Autodesk Inventor part; units mm, degrees
ref_plane "YZ Plane" through (0, 0, 0) normal (1, 0, 0) x (0, 1, 0)
ref_plane "XZ Plane" through (0, 0, 0) normal (0, 1, 0) x (-1, 0, 0)
ref_plane "XY Plane" through (0, 0, 0) normal (0, 0, 1) x (1, 0, 0)
sketch "Sketch1" plane through (0, 0, 0) normal (0, 0, 1) x (1, 0, 0)
  line L0 (-2, 0) -> (2, 0)
  line L1 (-2, 0) -> (-2, 3)
  line L2 (-2, 3) -> (-1.9, 3)
  line L3 (0, 0) -> (0, 3) construction
  line L4 (-1.9, 3) -> (-1.9, 3.6)
  line L5 (-1.5, 4) -> (-1.3196, 4)
  line L6 (-0.9732, 3.8) -> (-0.6268, 3.2)
  line L7 (-0.2804, 3) -> (0, 3)
  arc A0 (-0.9732, 3.8) -> (-1.3196, 4) centre (-1.3196, 3.6) ccw
  arc A1 (-0.6268, 3.2) -> (-0.2804, 3) centre (-0.2804, 3.4) ccw
  arc A2 (-1.5, 4) -> (-1.9, 3.6) centre (-1.5, 3.6) ccw
  line L8 (2, 0) -> (2, 3)
  line L9 (2, 3) -> (1.9, 3)
  line L10 (1.9, 3) -> (1.9, 3.6)
  line L11 (1.5, 4) -> (1.3196, 4)
  line L12 (0.9732, 3.8) -> (0.6268, 3.2)
  line L13 (0.2804, 3) -> (0, 3)
  arc A3 (1.3196, 4) -> (0.9732, 3.8) centre (1.3196, 3.6) ccw
  arc A4 (0.2804, 3) -> (0.6268, 3.2) centre (0.2804, 3.4) ccw
  arc A5 (1.9, 3.6) -> (1.5, 4) centre (1.5, 3.6) ccw
  line L14 (-0.8, 3.5) -> (0.8, 3.5) construction
  dimension "d0" = 0.4
  dimension "d1" = 8
  dimension "d2" = 6
  dimension "d3" = 6
  dimension "d4" = 4
  dimension "d5" = 3.8
  dimension "d8" = 1.6
  dimension "d9" = 120
revolve "Revolution1" add sketch "Sketch1" angle 360 about axis through (-2, 0, 0) along (1, 0, 0)
sketch "Sketch2" plane through (2, 0, 0) normal (1, 0, 0) x (0, 0, -1)
  circle A0 centre (0, 0) radius 2.5
  line L0 (2.2405, -1.1091) -> (1.6314, -0.5) construction
  line L1 (1.1314, 0) -> (1.6314, 0.5)
  line L2 (-2.2405, 1.1091) -> (-1.6314, 0.5) construction
  line L3 (-1.1314, 0) -> (-1.6314, -0.5)
  line L4 (-1.1091, -2.2405) -> (0, -1.1314)
  line L5 (0, -1.1314) -> (1.1091, -2.2405)
  line L6 (1.1091, 2.2405) -> (0, 1.1314)
  line L7 (0, 1.1314) -> (-1.1091, 2.2405)
  line L8 (-1.6314, -0.5) -> (-2.4495, -0.5)
  line L9 (-1.6314, 0.5) -> (-2.4495, 0.5)
  line L10 (1.6314, -0.5) -> (2.4495, -0.5)
  line L11 (1.6314, 0.5) -> (2.4495, 0.5)
  line L12 (-1.6314, -0.5) -> (-2.2405, -1.1091) construction
  line L13 (1.6314, -0.5) -> (1.1314, 0)
  line L14 (1.6314, 0.5) -> (2.2405, 1.1091) construction
  line L15 (-1.6314, 0.5) -> (-1.1314, 0)
  point P0 (0, 0)
  dimension "d11" = 5
  dimension "d12" = 1.6
  dimension "d13" = 1
  dimension "d14" = 1
  dimension "d15" = 1.5685
  dimension "d16" = 1.5685
  dimension "d17" = 1.6
  dimension "d18" = 1.6
  dimension "d19" = 1.6
extrude "Extrusion1" cut sketch "Sketch2" against normal through all contours L11 L1 L13 L10 A0 L5 L4 L8 L3 L15 L9 L7 L6
fillet "Fillet1" radius 0.3 6 edges at (0, 0, 1.1314) (0, 0.5, 1.6314) (0, -0.5, 1.6314) (0, 0.5, -1.6314) (0, 0, -1.1314) (0, -0.5, -1.6314)
fillet "Fillet2" radius 0.8 2 edges at (0, -1.1314, 0) (0, 1.1314, 0)
equation "\"d3\" = d2"
equation "\"d14\" = d13"
equation "\"d16\" = d15"
equation "\"d17\" = d12"
equation "\"d18\" = d17"
equation "\"d19\" = d12"
properties part number "4265C" material "Steel"
The listing builds one solid part. Answer for the finished solid, in the listing's coordinates (mm). A direction names the side the tool comes from. Round coordinates to 2 decimals unless told otherwise and drop trailing zeros. Put each result on its own line as item: value.
Q1. Which of the six approach directions +Z, -Z, +X, -X, +Y, -Y give full straight-line access (tool end or side, diameter ignored) to faces 1 (the flat face through (-1.9, -1, 3)), 2 (the cylindrical face through (-0.028, 1.463, -0.009)), 3 (the flat face through (-2, 0, -2))?
Results list:
face 1: -X
face 2: +X, -X
face 3: +Z, -Z, -X, +Y, -Y
Q2. Consider line 1 along Y through (x, z) = (-1.15, 2); line 2 along Z through (x, y) = (-0.65, 2); line 3 along Y through (x, z) = (0.75, 1.75). Determine where each line is inside the solid, lowest interval first.
Results list:
line 1: -3.42 to -1.5, -0.5 to 0.5, 1.5 to 3.42
line 2: -2.55 to -1.5, -0.87 to 0.87, 1.5 to 2.55
line 3: -2.93 to -1.79, -0.5 to 0.5, 1.79 to 2.93
Q3. Determine the mould class of faces 4 (the cylindrical face through (0, -1.5, 2)), 5 (the cylindrical face through (0, -3, 0)), 6 (the flat face through (1.9, -1, 3)) for opening direction Y: pulls with the +Y half, pulls with the -Y half, needs draft (parallel to the pull), parting line crosses it, or undercut.
Results list:
face 4: undercut
face 5: parting line crosses it
face 6: needs draft
Q4. Each of these flat-tipped pins is pushed along its axis until it touches: P1, Ø0.6, axis at x = 1, z = 2, coming from the -Y side; P2, Ø0.8, axis at x = 0, z = -2, coming from the +Y side; P3, Ø1.5, axis at x = 1.5, y = -1.5, coming from the -Z side. Where does it stop, or does it pass through?
Results list:
P1: y = -3.56
P2: y = 2.54
P3: z = -3.93
